Part print with two shaded views. Sizes in mm from the minimum x, y, z corner. Coordinates: 2 decimals unless noted, no trailing zeros. Order: outer loops, then holes, each group sorted by start corner. A loop starts at its lowest first (then second) coordinate and runs counter-clockwise, first axis right, second up. Notation, with made-up numbers: (11, -24) - (48, -24) arc R22 cw to (48, 3) - close; hole circle Ø11 at (19.25, -24.5). An arc over 180 degrees is marked (long way). Return JSON: item names as keys, results as strings.
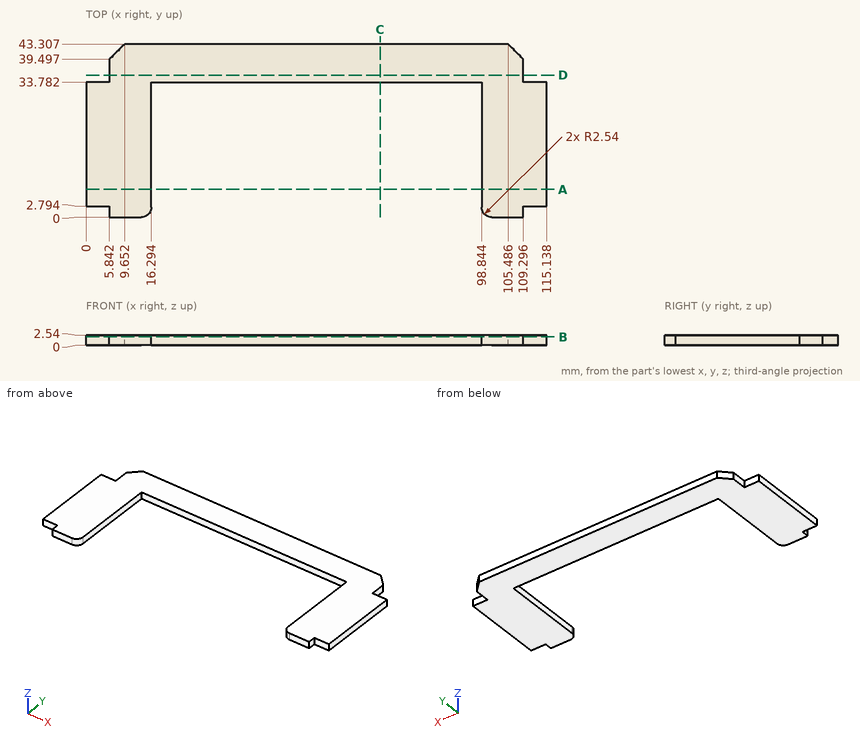
Item 1: Band-saw the part on D-D, the plane y = 35.5. List the corners of the cut face in (x, z).
Findings below:
{"outline": "(5.84, 0) - (109.3, 0) - (109.3, 2.54) - (5.84, 2.54) - close"}
Item 2: Drop flat-ended pins along their axis: P1, Ø0.8, axis at x = 112, z = 1.5, coming from the -Y side; P2, Ø1, axis at x = 35.5, z = 0.5, coming from the -Y side; P3, Ø0.8, axis at y = 1.5, z = 1, coming from the -X side. Give the stop position or say it passes through.
Findings below:
{"P1": "stops at y = 2.79", "P2": "stops at y = 33.78", "P3": "stops at x = 5.84"}
Item 3: Band-saw the part on A-A, the plane y = 7. List the corners of the cut face in (x, z).
Findings below:
{"outline": "(0, 0) - (16.29, 0) - (16.29, 2.54) - (0, 2.54) - close; (98.84, 0) - (115.14, 0) - (115.14, 2.54) - (98.84, 2.54) - close"}
Item 4: Wall check: L1, parallel to X at y = 10.5, z = 2.25; L2, parallel to Y at x = 24.5, z = 1.4; L3, parallel to X at y = 36, z = 2.4. Give the ranges that are in metal, low to high. Write a range as [from, to].
Findings below:
{"L1": "x = [0, 16.29], [98.84, 115.14]", "L2": "y = [33.78, 43.31]", "L3": "x = [5.84, 109.3]"}
Item 5: Band-saw the part on C-C, the plane x = 73.5. List the corners of the cut face in (y, z), then the cut area to 3 significant figures.
Findings below:
{"outline": "(33.78, 0) - (43.31, 0) - (43.31, 2.54) - (33.78, 2.54) - close", "area": "24.2 mm²"}
Item 6: Band-saw the part on B-B, the plane z = 2.15. List the corners of the cut face in (x, y).
Findings below:
{"outline": "(0, 2.79) - (5.84, 2.79) - (5.84, 0) - (13.75, 0) arc R2.54 ccw to (16.29, 2.54) - (16.29, 33.78) - (98.84, 33.78) - (98.84, 2.54) arc R2.54 ccw to (101.38, 0) - (109.3, 0) - (109.3, 2.79) - (115.14, 2.79) - (115.14, 33.78) - (109.3, 33.78) - (109.3, 39.5) - (105.49, 43.31) - (9.65, 43.31) - (5.84, 39.5) - (5.84, 33.78) - (0, 33.78) - close"}
